Build history of the part. All positions in model axes, mm. Face numbers are marked on the shaded views. Coordinates: 2 decimals unless noted, no trailing zeros. Loops run counter-clockwise (first coordinate to the right, second up) from the corner with the lowest first, then second, coordinate; pieces in that order, holes last.
(1) Slice it at A-A (y = 11). Give the number of separate pieces and of enclosed holes in the cut face, and give its area (3 significant figures).
(2) Flat gauge pins, fed straight in: P1, Ø6.5, axis at x = -11, y = 11, coming from the +Z side; P2, Ø1, axis at y = 0, z = 1.5, coming from the +X side; P3, Ø3.5, axis at x = -11, y = 10, coming from the +Z side. Where does each tip first touch, or does it go through?
(3) Wall check: L1, parallel to Y at x = 11, z = 1.9; L2, parallel to X at y = -11, z = 2; L3, parallel to X at y = 11, z = 1.8. Give the ranges that are in metal, low to high.
(4) Two-plate mould, pull along X, no slides. Class the marked faces 1, 2 and 3: pulls with the +X half, pulls with the -X half, needs draft (parallel to the pull), parting line crosses it, or undercut.
(5) Slice it at C-C (y = 2.5). Give the cut face in (x, z), and give its area (3 significant figures).
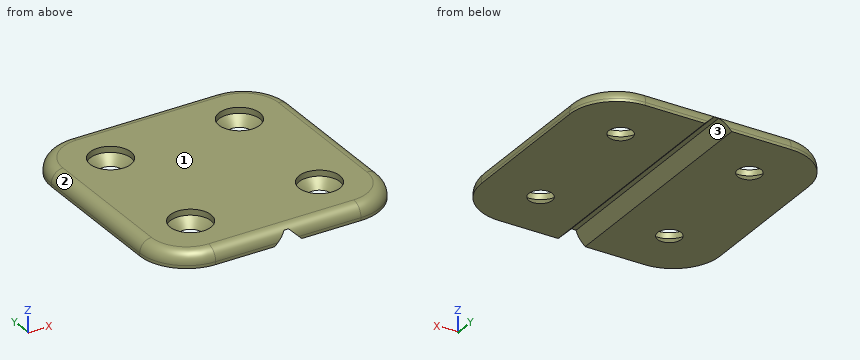
from build123d import *

# Parameters (mm, degrees)
F0_R     = 3.5
F0_R_2   = 2
F1_DEPTH = 1.5
F2_DEPTH = 2.5
F3_R     = 2
F4_SIZE  = 1.49999
F7_DEPTH = 40.301


# Not quite as in the source:
# - a fillet or chamfer is up to 0.001 mm smaller than in the source, because OpenCascade refuses the exact size


with BuildPart() as f1:
    # F0 (on Top) → F1 (new body)
    with BuildSketch(Plane.XY):
        with BuildLine():
            ThreePointArc((20.4, 12.15), (18.0568542495, 17.8068542495), (12.4, 20.15))
            Line((12.4, 20.15), (-12.4, 20.15))
            ThreePointArc((-12.4, 20.15), (-18.0568542495, 17.8068542495), (-20.4, 12.15))
            Line((-20.4, 12.15), (-20.4, -12.15))
            ThreePointArc((-20.4, -12.15), (-18.0568542495, -17.8068542495), (-12.4, -20.15))
            Line((-12.4, -20.15), (12.4, -20.15))
            ThreePointArc((12.4, -20.15), (18.0568542495, -17.8068542495), (20.4, -12.15))
            Line((20.4, -12.15), (20.4, 12.15))
        make_face()
        with Locations((-11, -11)):
            Circle(F0_R, mode=Mode.SUBTRACT)
        with Locations((11, -11)):
            Circle(F0_R, mode=Mode.SUBTRACT)
        with Locations((-11, 11)):
            Circle(F0_R, mode=Mode.SUBTRACT)
        with Locations((11, 11)):
            Circle(F0_R, mode=Mode.SUBTRACT)
        with Locations((-11, 11)):
            Circle(F0_R)
        with Locations((-11, 11)):
            Circle(F0_R_2, mode=Mode.SUBTRACT)
        with Locations((11, 11)):
            Circle(F0_R)
        with Locations((11, 11)):
            Circle(F0_R_2, mode=Mode.SUBTRACT)
        with Locations((11, -11)):
            Circle(F0_R)
        with Locations((11, -11)):
            Circle(F0_R_2, mode=Mode.SUBTRACT)
        with Locations((-11, -11)):
            Circle(F0_R)
        with Locations((-11, -11)):
            Circle(F0_R_2, mode=Mode.SUBTRACT)
    extrude(amount=F1_DEPTH)

    # F0 (on Top) → F2 (join)
    with BuildSketch(Plane.XY):
        with BuildLine():
            ThreePointArc((20.4, 12.15), (18.0568542495, 17.8068542495), (12.4, 20.15))
            Line((12.4, 20.15), (-12.4, 20.15))
            ThreePointArc((-12.4, 20.15), (-18.0568542495, 17.8068542495), (-20.4, 12.15))
            Line((-20.4, 12.15), (-20.4, -12.15))
            ThreePointArc((-20.4, -12.15), (-18.0568542495, -17.8068542495), (-12.4, -20.15))
            Line((-12.4, -20.15), (12.4, -20.15))
            ThreePointArc((12.4, -20.15), (18.0568542495, -17.8068542495), (20.4, -12.15))
            Line((20.4, -12.15), (20.4, 12.15))
        make_face()
        with Locations((-11, -11)):
            Circle(F0_R, mode=Mode.SUBTRACT)
        with Locations((11, -11)):
            Circle(F0_R, mode=Mode.SUBTRACT)
        with Locations((-11, 11)):
            Circle(F0_R, mode=Mode.SUBTRACT)
        with Locations((11, 11)):
            Circle(F0_R, mode=Mode.SUBTRACT)
    extrude(amount=F2_DEPTH)

    # F3
    f3_edges = [f1.edges().sort_by_distance(p)[0] for p in [
        (-18.056854, 17.806854, 2.5),
    ]]
    fillet(f3_edges, radius=F3_R)

    # F4 (size 1.5 in the source; OpenCascade refuses exactly that, so slightly less here)
    f4_edges = [f1.edges().sort_by_distance(p)[0] for p in [
        (-13, 11, 1.5),
        (9, 11, 1.5),
        (9, -11, 1.5),
        (-13, -11, 1.5),
    ]]
    chamfer(f4_edges, length=F4_SIZE)

    # F6 (on offset) → F7 (cut, through all)
    with BuildSketch(Plane.XZ.offset(20.15)):
        Polygon((-0.4, 1.9), (-2.3, 0), (2.3, 0), (0.4, 1.9), align=None)
    extrude(amount=-F7_DEPTH, mode=Mode.SUBTRACT)


solid = f1.part
Response values:
1. separate pieces: 3
1. enclosed holes: 0
1. area: 64.7 mm2
2. P1: stops at z = 1.25
2. P2: stops at x = 20.34
2. P3: stops at z = 0.75
3. L1: y = -19.58 to -14.5, -7.5 to 7.5, 14.5 to 19.58
3. L2: x = -19.72 to -14.5, -7.5 to 7.5, 14.5 to 19.72
3. L3: x = -19.92 to -14.5, -7.5 to -0.5, 0.5 to 7.5, 14.5 to 19.92
4. face 1: needs draft
4. face 2: pulls with the -X half
4. face 3: undercut
5. outline: (-20.4, 0) - (-2.3, 0) - (-0.4, 1.9) - (0.4, 1.9) - (2.3, 0) - (20.4, 0) - (20.4, 0.5) arc R2 ccw to (18.4, 2.5) - (-18.4, 2.5) arc R2 ccw to (-20.4, 0.5) - close
5. area: 95.2 mm2
